Part model, mm, in its own coordinate system. A direction names the side the tool comes from. Round coordinates to 2 decimals unless told otherwise and drop trailing zeros. Loops run counter-clockwise (first coordinate to the right, second up) from the corner with the lowest first, then second, coordinate; pieces in that order, holes last.
from build123d import *

# Parameters (mm, degrees)
SKETCH2_R           = 25.4
BOSS_EXTRUDE1_DEPTH = 158.75
CUT_EXTRUDE1_DEPTH  = 47.625
SKETCH4_R           = 12.7
CUT_EXTRUDE2_DEPTH  = 48.625


with BuildPart() as part:
    # Sketch2 → Boss-Extrude1 (new body, symmetric)
    with BuildSketch(Plane(origin=(0, 0, 0), x_dir=(0, 0, -1), z_dir=(1, 0, 0))):
        Circle(SKETCH2_R)
    extrude(amount=BOSS_EXTRUDE1_DEPTH, both=True)

    # Sketch3 → Cut-Extrude1 (cut)
    with BuildSketch(Plane(origin=(158.75, 0, 0), x_dir=(0, 0, -1), z_dir=(1, 0, 0))):
        with BuildLine():
            Line((-22.225, 12.296722124), (-22.225, -12.296722124))
            ThreePointArc((-22.225, -12.296722124), (-25.4, 0), (-22.225, 12.296722124))
        make_face()
        with BuildLine():
            Line((22.225, 12.296722124), (22.225, -12.296722124))
            ThreePointArc((22.225, -12.296722124), (25.4, 0), (22.225, 12.296722124))
        make_face()
    extrude(amount=-CUT_EXTRUDE1_DEPTH, mode=Mode.SUBTRACT)

    # Sketch4 → Cut-Extrude2 (cut, through all)
    with BuildSketch(Plane.XY.offset(22.225)):
        with Locations((139.7, 0)):
            Circle(SKETCH4_R)
    extrude(amount=-CUT_EXTRUDE2_DEPTH, mode=Mode.SUBTRACT)


solid = part.part
1) Slice it at C-C, the plane x = -47. Give the cut face in (y, z).
Values:
outline: circle Ø50.8 at (0, 0)
2) Tool access for faces 4 (the face through (154, 0, -22.225)), 5 (the face through (158.75, 0, 0)), 6 (the face through (121, 0, 22.225)): list every direction of +Z, -Z, +X, -X, +Y, -Y with a clear straight run to the whole face (end or side of a thin tool).
Values:
face 4: -Z, +X, +Y, -Y
face 5: +Z, -Z, +X, +Y, -Y
face 6: +Z, +X, +Y, -Y
3) Mould opens along X. For faces 1 (the face through (-158.75, 0, 0)), 2 (the face through (151.814, 3.815, 0.311)), 3 (the face through (154, 0, 22.225)) say: released by +X, released by -X, zero draft, split by the parting line, or undercut.
Values:
face 1: released by -X
face 2: undercut
face 3: zero draft
4) Wall check: line 1 along X through (y, z) = (0, 2); line 2 along Y through (x, z) = (139, 12); line 3 along Y through (x, z) = (139.7, 2). Give the ranges that are in metal, low to high.
Values:
line 1: x = -158.75 to 127, 152.4 to 158.75
line 2: y = -22.39 to -12.68, 12.68 to 22.39
line 3: y = -25.32 to -12.7, 12.7 to 25.32
5) Drop flat-ended pins along their axis: pin 1 Ø8 at (x, y) = (-51, 4) entering from +Z; pin 2 Ø1.6 at (y, z) = (-5, 24) entering from +X (3 decimals); pin 3 Ø17.5 at (x, y) = (150.5, 0.5) entering from -Z (3 decimals); pin 4 Ø3 at (x, z) = (81.5, 4) entering from -Y. Give the stop position or say it passes through.
Values:
pin 1: stops at z = 25.4
pin 2: stops at x = 111.125
pin 3: stops at z = -22.225
pin 4: stops at y = -25.28
6) Slice it at A-A, the plane y = 0. Give the cut face in (x, z) (3 decimals).
Values:
outline: (-158.75, -25.4) - (111.125, -25.4) - (111.125, -22.225) - (127, -22.225) - (127, 22.225) - (111.125, 22.225) - (111.125, 25.4) - (-158.75, 25.4) - close; (152.4, -22.225) - (158.75, -22.225) - (158.75, 22.225) - (152.4, 22.225) - close
7) Slice it at B-B, the plane z = 0. Give the cut face in (x, y), then the cut area to 3 significant figures.
Values:
outline: (-158.75, -25.4) - (158.75, -25.4) - (158.75, 25.4) - (-158.75, 25.4) - close; hole circle Ø25.4 at (139.7, 0)
area: 15,600 mm2
8) Slice it at D-D, the plane x = 139.7. Give the cut face in (y, z).
Values:
outline: (-12.7, -22) - (-12.7, 22) arc R25.4 ccw to start; (12.7, -22) arc R25.4 ccw to (12.7, 22) - close
